Input: part model. Units: mm. Frame: model coordinates. A direction names the side the tool comes from. Coordinates: 2 decimals unless noted, no trailing zeros. Loops run counter-clockwise (first coordinate to the right, second up) from the corner with the lowest first, then second, coordinate; pieces in that order, holes last. Notation, with made-up numbers: (6, -35) -> (22, -35) arc R28 cw to (22, -4) -> close; hole circle Ø2 at (81.25, 41.25). An arc over 180 degrees is marked (long way). Answer as a JSON object with one key per item and string values.
Autodesk Inventor part; units mm, degrees
ref_plane "Work Plane2" through (0, 0, 0) normal (0.9999, 0, -0.0105) x (0, 1, 0)
ref_plane "YZ Plane" through (0, 0, 0) normal (1, 0, 0) x (0, 1, 0)
ref_plane "XZ Plane" through (0, 0, 0) normal (0, 1, 0) x (-1, 0, 0)
sketch "Sketch1" plane through (0, 0, 0) normal (0, 0, 1) x (1, 0, 0)
  circle A0 centre (0, 0) radius 12.7
  dimension "d0" = 25.4
extrude "Extrusion1" add sketch "Sketch1" along normal mid plane 107.6
shell "Shell1" thickness 1.65 removed faces 2 at (-3.6254, -0.9542, 53.8) at (-3.6254, -0.9542, -53.8)
ref_plane "Work Plane2" through (0, 0, 0) normal (0.9999, 0, -0.0105) x (0, 1, 0)
sketch "Sketch6" plane through (0, 0, 0) normal (0.9999, 0, -0.0105) x (0, 1, 0)
  ellipse E0 centre (0, -53.7971) end of major axis (-12.7, -53.7971) minor radius 0.133
  ellipse E1 centre (0, 53.7971) end of major axis (12.7, 53.7971) minor radius 0.133
  line L0 (0, -53.7971) -> (0, 53.7971) construction
  circle A0 centre (0, 0) radius 12.7
  circle A1 centre (0, 0) radius 11.05
  dimension "d19" = 25.4
  dimension "d20" = 1.65
extrude "Extrusion3" add sketch "Sketch6" along normal blind 53.8 contours A0
properties part number "EQ TEE (ASME BPE - 89.4 or 90.6 DEG)-25.4"
1. Mould query, pull axis Z, two halves, no side actions, for faces 3 (the face through (-1, -11.2, -53.8)), 4 (the face through (4.15, 0.24, -11.09)), 5 (the face through (-11.04, -0.49, -0.75)). Classes: pulls with the +Z half, pulls with the -Z half, needs draft (parallel to the pull), parting line crosses it, or undercut.
Reply:
{"face 3": "pulls with the -Z half", "face 4": "undercut", "face 5": "needs draft"}
2. Pin query (flat end, axial travel): P1, Ø2, axis at x = 26.5, z = -3, coming from the +Y side; P2, Ø8, axis at x = 44, y = 3.5, coming from the -Z side; P3, Ø12, axis at y = -10, z = 12.5, coming from the -X side. Return the tip coordinate at first contact, or that it passes through.
Reply:
{"P1": "stops at y = 12.58", "P2": "stops at z = -13.18", "P3": "stops at x = -12.05"}
3. Access query for faces 1 (the face through (4.292, -0.243, 11.003)), 2 (the face through (-1, -11.2, 53.8)). Directions: +Z, -Z, +X, -X, +Y, -Y. A direction counts if a zero-diameter tool reaches every point of the face in a straight line with its end or side. Return the directions, or none.
Reply:
{"face 1": "none", "face 2": "+Z, +X, -X, +Y, -Y"}
4. Line query: line 1 along Y through (x, z) = (0, 4); line 2 along X through (y, z) = (2.5, -45); line 3 along Z through (x, y) = (43, -5.25). Output: solid intervals per line, ascending.
Reply:
{"line 1": "y = -12.7 to -11.05, 11.05 to 12.7", "line 2": "x = -12.45 to -10.76, 10.76 to 12.45", "line 3": "z = -12.02 to -10.18, 9.27 to 11.11"}
5. Section query B-B (x = -8). Return loops of the section in (y, z), plus the area to 3 significant figures.
Reply:
{"outline": "(-9.86, -53.8) -> (-7.62, -53.8) -> (-7.62, 53.8) -> (-9.86, 53.8) -> close; (7.62, -53.8) -> (9.86, -53.8) -> (9.86, 53.8) -> (7.62, 53.8) -> close", "area": "482 mm2"}
6. Section query D-D (y = -8). Return loops of the section in (x, z).
Reply:
{"outline": "(-9.86, -53.8) -> (-7.62, -53.8) -> (-7.62, 53.8) -> (-9.86, 53.8) -> close; (-0.1, -9.86) -> (7.62, -9.94) -> (7.62, -53.8) -> (9.86, -53.8) -> (9.86, -9.97) -> (53.69, -10.43) -> (53.72, -8.19) -> (9.86, -7.73) -> (9.86, 7.52) -> (53.88, 7.06) -> (53.9, 9.3) -> (9.86, 9.76) -> (9.86, 53.8) -> (7.62, 53.8) -> (7.62, 9.78) -> (0.1, 9.86) -> (0.08, 7.62) -> (7.62, 7.54) -> (7.62, -7.7) -> (-0.08, -7.62) -> close"}
7. Section query A-A (y = 3). Return loops of the section in (x, z).
Reply:
{"outline": "(-12.34, -53.8) -> (-10.63, -53.8) -> (-10.63, 53.8) -> (-12.34, 53.8) -> close; (-0.13, -12.34) -> (10.63, -12.45) -> (10.63, -53.8) -> (12.34, -53.8) -> (12.34, -12.47) -> (53.67, -12.9) -> (53.69, -11.2) -> (12.34, -10.77) -> (12.34, 10.51) -> (53.91, 10.07) -> (53.93, 11.77) -> (12.34, 12.21) -> (12.34, 53.8) -> (10.63, 53.8) -> (10.63, 12.23) -> (0.13, 12.34) -> (0.11, 10.63) -> (10.63, 10.52) -> (10.63, -10.75) -> (-0.11, -10.63) -> close"}
8. Section query C-C (z = -30.5). Return loops of the section in (x, y).
Reply:
{"outline": "circle Ø25.4 at (0, 0); hole circle Ø22.1 at (0, 0)"}
